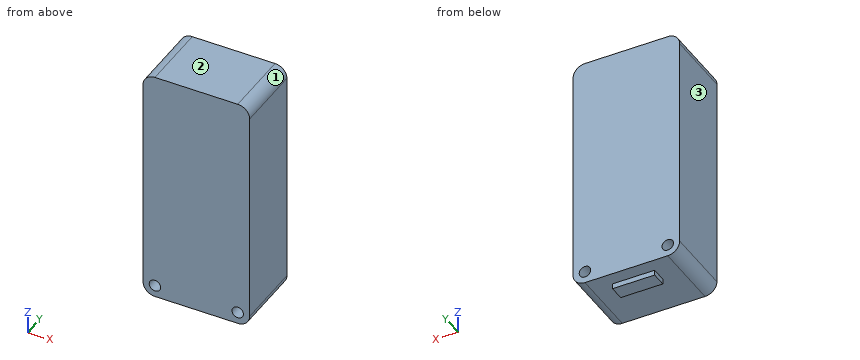
from build123d import *

# Parameters (mm, degrees)
SKETCH1_W               = 22.76
SKETCH1_H               = 51.13
BOSS_EXTRUDE1_DEPTH     = 14.62
CUT_EXTRUDE1_DEPTH      = 58.844955701
CUT_EXTRUDE1_DEPTH_BACK = 58.844955701
SKETCH2_R               = 1.225
FILLET1_R               = 2.54
SKETCH4_W               = 9
SKETCH4_H               = 3.2
BOSS_EXTRUDE3_DEPTH     = 1.12


with BuildPart() as part:
    # Sketch1 → Boss-Extrude1 (new body)
    with BuildSketch(Plane(origin=(0, 0, 0), x_dir=(1, 0, 0), z_dir=(0, 1, 0))):
        with Locations((11.38, -25.565)):
            Rectangle(SKETCH1_W, SKETCH1_H)
    extrude(amount=BOSS_EXTRUDE1_DEPTH)

    # Sketch2 → Cut-Extrude1 (cut, two sides: drawn at the far end of the back side and taken through both)
    with BuildSketch(Plane(origin=(0, 14.62, 0), x_dir=(1, 0, 0), z_dir=(0, 1, 0)).offset(-CUT_EXTRUDE1_DEPTH_BACK)):
        with Locations(Location((2.54, -2.54, 0), (0, 0, 270))):
            Circle(SKETCH2_R)
        with Locations(Location((20.22, -2.54, 0), (0, 0, 270))):
            Circle(SKETCH2_R)
    extrude(amount=CUT_EXTRUDE1_DEPTH + CUT_EXTRUDE1_DEPTH_BACK, mode=Mode.SUBTRACT)

    # Fillet1
    fillet1_edges = [part.edges().sort_by_distance(p)[0] for p in [
        (0, 7.31, 0),
        (22.76, 7.31, 0),
        (22.76, 7.31, 51.13),
        (0, 7.31, 51.13),
    ]]
    fillet(fillet1_edges, radius=FILLET1_R)

    # Sketch4 → Boss-Extrude3 (add)
    with BuildSketch(Plane(origin=(0, 0, 0), x_dir=(-1, 0, 0), z_dir=(0, 0, -1))):
        with Locations((-11.38, 10.19)):
            Rectangle(SKETCH4_W, SKETCH4_H)
    extrude(amount=BOSS_EXTRUDE3_DEPTH)


solid = part.part
The model under review builds one solid part; all positions refer to its coordinate system, in mm. Face numbers are marked on the shaded views. Give positions to 0.01 mm unless a question says otherwise; leave off trailing zeros. Write each loop counter-clockwise with the first axis right and the second up, starting at its lowest first coordinate (ties: lowest second). Pieces come first, ordered by that corner, then holes.
1. Draft analysis for pull direction X (two halves, no side actions). For the marked faces 1, 2 and 3, state which applies: +X half, -X half, draft (parallel to the pull), parting line (faces both ways), or undercut.
2. Add section B-B, the plane x = 12. Write out the cut boundary in (y, z), plus the area to 3 significant figures.
3. Wall thickness on L1, parallel to X at y = 9.75, z = 2.54 (3 decimals); L2, parallel to X at y = 14.25, z = 3.5; L3, parallel to Z at x = 20.5, y = 11.25: over which ranges is each line inside the solid? List them lowest first.
4. Add section A-A, the plane y = 13.5. Write out the cut boundary in (x, z) (3 decimals), plus the area to 3 significant figures.
5. For P1, Ø0.6, axis at x = 12, z = -0.5, coming from the +Y side, flat-tipped, find the tip position at first contact; note if it passes through.
6. Add section C-C, the plane x = 17.5. Write out the cut boundary in (y, z).
Worked answers:
1. face 1: +X half
1. face 2: draft
1. face 3: -X half
2. outline: (0, 0) - (8.59, 0) - (8.59, -1.12) - (11.79, -1.12) - (11.79, 0) - (14.62, 0) - (14.62, 51.13) - (0, 51.13) - close
2. area: 751 mm2
3. L1: x = 0 to 1.315, 3.765 to 18.995, 21.445 to 22.76
3. L2: x = 0 to 1.78, 3.3 to 19.46, 20.98 to 22.76
3. L3: z = 0.02 to 1.35, 3.73 to 51.11
4. outline: (0, 2.54) arc R2.54 ccw to (2.54, 0) - (20.22, 0) arc R2.54 ccw to (22.76, 2.54) - (22.76, 48.59) arc R2.54 ccw to (20.22, 51.13) - (2.54, 51.13) arc R2.54 ccw to (0, 48.59) - close; hole circle Ø2.45 at (2.54, 2.54); hole circle Ø2.45 at (20.22, 2.54)
4. area: 1,150 mm2
5. P1: stops at y = 11.79
6. outline: (0, 0) - (14.62, 0) - (14.62, 51.13) - (0, 51.13) - close
